Source: CAD feature listing. Evaluate the final solid. Frame: model axes, mm. Round coordinates to 2 decimals unless told otherwise and drop trailing zeros. Loops run counter-clockwise (first coordinate to the right, second up) from the corner with the lowest first, then second, coordinate; pieces in that order, holes last. Notation, with made-up numbers: (-5.5, 32) - (40.5, 32) arc R24 ccw to (40.5, 44) - close; hole circle Ø2 at (1, 14.25). An arc over 180 degrees is marked (long way). One line per question, with ' | ' between items.
from build123d import *

# Parameters (mm, degrees)
F0_W      = 50
F0_H      = 100
F1_DEPTH  = 5
F2_W      = 30
F2_H      = 2
F3_DEPTH  = 45
F5_DEPTH  = 41
F6_W      = 0.475269
F6_H      = 150
F7_DEPTH  = 1
F7_FACE_W = 0.47527
F7_FACE_H = 1
F8_DEPTH  = 30


with BuildPart() as f1:
    # F0 (on Front) → F1 (new body)
    with BuildSketch(Plane.XZ):
        with Locations((-10.973271, -9.118421)):
            Rectangle(F0_W, F0_H)
    extrude(amount=F1_DEPTH)

    # F2 (on face) → F3 (join)
    with BuildSketch(Plane.XZ.offset(5)):
        with Locations((-10.973271, -1)):
            Rectangle(F2_W, F2_H)
    extrude(amount=F3_DEPTH)

    # F4 (on face) → F5 (cut)
    with BuildSketch(Plane(origin=(0, 0, -2), x_dir=(1, 0, 0), z_dir=(0, 0, -1))):
        Polygon((-24.382181, 5), (-21.973271, 5), (0, 5), (2.364369, 5), (2.364369, 48.887726), (-24.382181, 48.887726), align=None)
    extrude(amount=-F5_DEPTH, mode=Mode.SUBTRACT)

    # F6 (on face) → F7 (join)
    with BuildSketch(Plane.XY):
        with Locations((2.854673, -87.759547)):
            Rectangle(F6_W, F6_H)
    extrude(amount=F7_DEPTH)

    # F7_face (on face) → F8 (join)
    with BuildSketch(Plane(origin=(2.854674, -162.759547, 0.5), x_dir=(1, 0, 0), z_dir=(0, -1, 0))):
        Rectangle(F7_FACE_W, F7_FACE_H)
    extrude(amount=F8_DEPTH)


solid = f1.part
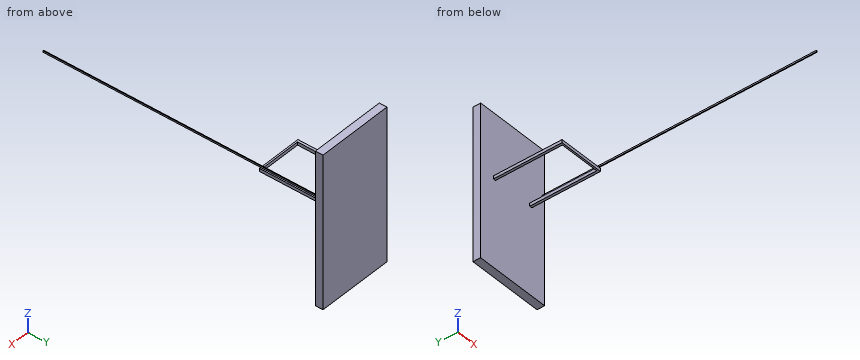
1. Material intervals for probe 1 along Y at (x, z) = (-14.5, -28), sorted ascending.
Worked out:
probe 1: y = -5 to 0
2. Contact query for flat-ended pins moving along their axis: P1, Ø0.5, axis at x = 3, y = -105.5, coming from the -Z side; P2, Ø1, axis at x = -16.5, z = -1.5, coming from the -Y side; P3, Ø5, axis at x = -11.5, z = 26.5, coming from the -Y side. Output: stop coordinate, or through.
Worked out:
P1: stops at z = 0 | P2: stops at y = -50 | P3: stops at y = -5
3. Section query B-B, the plane y = -38.5. Return loops of the section in (x, z), plus the area to 3 significant figures.
Worked out:
outline: (-25.97, -2) - (-24.38, -2) - (-24.38, 0) - (-25.97, 0) - close; (2.36, -2) - (4.03, -2) - (4.03, 0) - (3.09, 0) - (3.09, 1) - (2.62, 1) - (2.62, 0) - (2.36, 0) - close | area: 6.98 mm2
4. Section query C-C, the plane y = -60.5. Return loops of the section in (x, z), plus the area to 3 significant figures.
Worked out:
outline: (2.62, 0) - (3.09, 0) - (3.09, 1) - (2.62, 1) - close | area: 0.475 mm2
5. Section query D-D, the plane z = -4.5. Return loops of the section in (x, y), plus the area to 3 significant figures.
Worked out:
outline: (-35.97, -5) - (14.03, -5) - (14.03, 0) - (-35.97, 0) - close | area: 250 mm2
6. Section query A-A, the plane x = -1.5. Return loops of the section in (y, z), plus the area to 3 significant figures.
Worked out:
outline: (-50, -2) - (-48.89, -2) - (-48.89, 0) - (-50, 0) - close; (-5, -59.12) - (0, -59.12) - (0, 40.88) - (-5, 40.88) - close | area: 502 mm2
